The listing builds one solid part. Answer for the finished solid, in the listing's coordinates (mm). Coordinates: 2 decimals unless noted, no trailing zeros. Order: outer loops, then holes, each group sorted by start corner. A loop starts at its lowest first (then second) coordinate and runs counter-clockwise, first axis right, second up. Notation, with made-up numbers: (14.5, 12.25) -> (60.5, 12.25) arc R18 cw to (60.5, 16.25) -> close; hole circle Ø7 at (-30, -11.5). An arc over 180 degrees is marked (long way). One line per question, with ' | ' between items.
from build123d import *

# Parameters (mm, degrees)
SKETCH_1_W             = 19.3
SKETCH_1_H             = 2
SM_BASE_FLANGE_1_DEPTH = 46.3
SKETCH_7_R             = 2.3
CUT_EXTRUDE_2_DEPTH    = 51.201394403
CHAMFER_2_SIZE         = 2.05


# Sheet-metal steps are written as plain solids
with BuildPart() as part:
    # Sketch 1 → Базовая кромка1 (new body)
    with BuildSketch(Plane(origin=(0, 0, 0), x_dir=(0, 0, -1), z_dir=(1, 0, 0))):
        with Locations((9.65, 1)):
            Rectangle(SKETCH_1_W, SKETCH_1_H)
    extrude(amount=-SM_BASE_FLANGE_1_DEPTH)

    # Эскиз7 → Вырез-Вытянуть2 (cut, through all)
    with BuildSketch(Plane(origin=(0, 2, 0), x_dir=(1, 0, 0), z_dir=(0, 1, 0))):
        with Locations(Location((-8, 9.3, 0), (0, 0, 270))):
            Circle(SKETCH_7_R)
    extrude(amount=-CUT_EXTRUDE_2_DEPTH, mode=Mode.SUBTRACT)

    # Фаска2
    # the kernel refuses this chamfer: 2.05 mm, written as the material it takes off along each edge
    with BuildSketch(Plane(origin=(-8, 0, -9.3), x_dir=(0, 0, 1), z_dir=(-1, 0, 0))) as chamfer_2_piece_1:
        Polygon((2.3 + CHAMFER_2_SIZE, 0), (2.3, CHAMFER_2_SIZE), (2.3, 0), align=None)
    revolve(axis=Axis((-8, 0, -9.3), (0, 1, 0)), mode=Mode.SUBTRACT)


solid = part.part
Item 1: Section B-B, the plane y = 0.9 is taken. Give the vertices of the cut face in (x, z).
Computed values:
outline: (-46.3, -19.3) -> (0, -19.3) -> (0, 0) -> (-46.3, 0) -> close; hole circle Ø6.9 at (-8, -9.3)
Item 2: Find the intervals of material crossed by L1, parallel to X at y = 0.9, z = -7.5; L2, parallel to X at y = 0.8, z = -9.25; L3, parallel to Z at x = -7, y = 1.4, in increasing order.
Computed values:
L1: x = -46.3 to -10.94, -5.06 to 0 | L2: x = -46.3 to -11.55, -4.45 to 0 | L3: z = -19.3 to -12.08, -6.52 to 0
Item 3: Section C-C, the plane x = -8 is taken. Give the vertices of the cut face in (y, z), plus the area to 3 significant figures.
Computed values:
outline: (0, -19.3) -> (2, -19.3) -> (2, -11.65) -> (0, -13.65) -> close; (0, -4.95) -> (2, -6.95) -> (2, 0) -> (0, 0) -> close | area: 25.2 mm^2
Item 4: Section A-A, the plane z = -9.3 is taken. Give the vertices of the cut face in (x, y), plus the area to 3 significant figures.
Computed values:
outline: (-46.3, 0) -> (-12.35, 0) -> (-10.35, 2) -> (-46.3, 2) -> close; (-5.65, 2) -> (-3.65, 0) -> (0, 0) -> (0, 2) -> close | area: 79.2 mm^2
